Part print with two shaded views. Sizes in mm from the minimum x, y, z corner. Round coordinates to 2 decimals unless told otherwise and drop trailing zeros. Order: outer loops, then holes, each group sorted by start corner. A loop starts at its lowest first (then second) coordinate and runs counter-clockwise, first axis right, second up. Notation, with made-up numbers: M 64,16 L 71,16 A16 cw 71,30 Z; hole C 56,42.5 d1. An arc over 180 degrees is marked long. One line per question, with ' | ' between items. Start each with the question number.
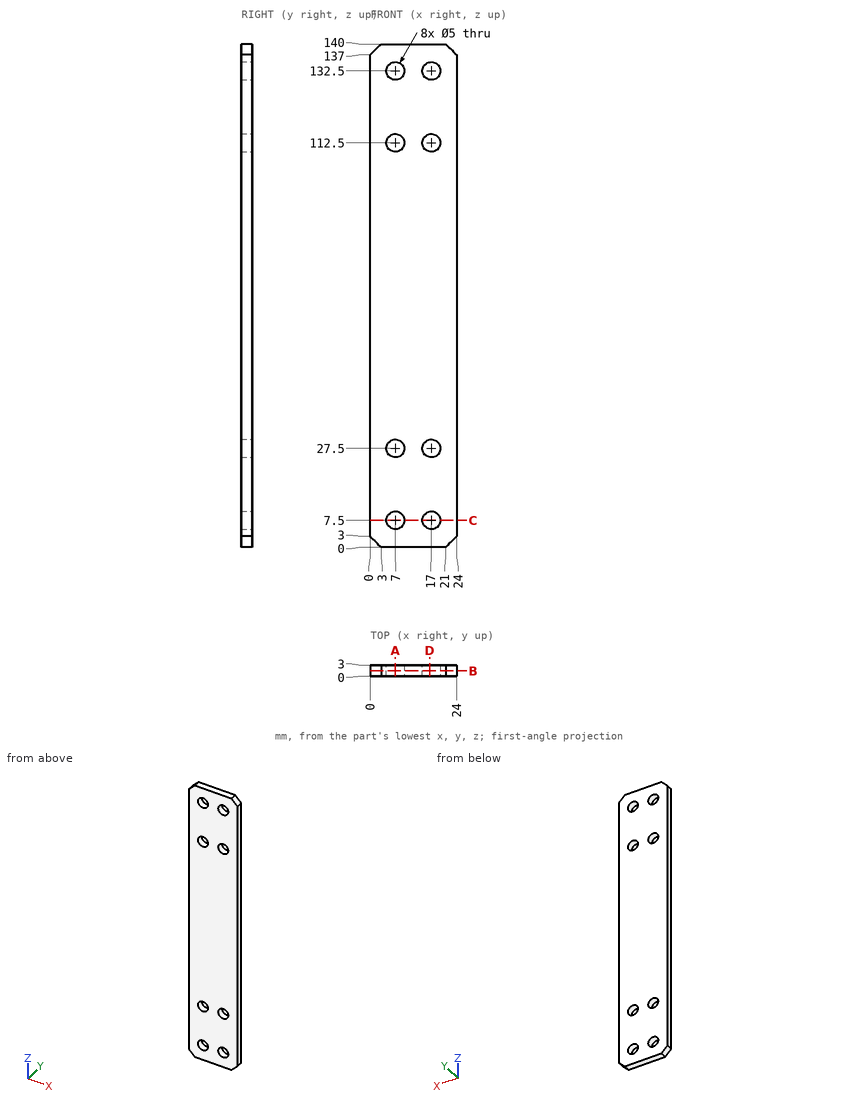
Item 1: Cut at D-D on x = 16.5. Write the cut outline in (y, z).
Item 2: Wall check: line 1 along X through (y, z) = (2.15, 27.5); line 2 along Z through (x, y) = (17, 0.65); line 3 along Z through (x, y) = (6.5, 1.6). Give the ranges that are in metal, low to high. Write a range as [from, to].
Item 3: Cut at C-C on z = 7.5. Write the cut outline in (x, y), then the cut area to 3 significant figures.
Item 4: Cut at B-B on y = 1.45. Count the separate pieces of the cut face and the enclosed holes in it, then the cut area to 3 significant figures.
Item 5: Cut at A-A on x = 7. Write the cut outline in (y, z), then the cut area to 3 significant figures.
Results found:
1) outline: M 0,0 L 3,0 L 3,5.05 L 0,5.05 Z; M 0,9.95 L 3,9.95 L 3,25.05 L 0,25.05 Z; M 0,29.95 L 3,29.95 L 3,110.05 L 0,110.05 Z; M 0,114.95 L 3,114.95 L 3,130.05 L 0,130.05 Z; M 0,134.95 L 3,134.95 L 3,140 L 0,140 Z
2) line 1: x = [0, 4.5], [9.5, 14.5], [19.5, 24] | line 2: z = [0, 5], [10, 25], [30, 110], [115, 130], [135, 140] | line 3: z = [0, 5.05], [9.95, 25.05], [29.95, 110.05], [114.95, 130.05], [134.95, 140]
3) outline: M 0,0 L 4.5,0 L 4.5,3 L 0,3 Z; M 9.5,0 L 14.5,0 L 14.5,3 L 9.5,3 Z; M 19.5,0 L 24,0 L 24,3 L 19.5,3 Z | area: 42.0 mm^2
4) separate pieces: 1 | enclosed holes: 8 | area: 3,180 mm^2
5) outline: M 0,0 L 3,0 L 3,5 L 0,5 Z; M 0,10 L 3,10 L 3,25 L 0,25 Z; M 0,30 L 3,30 L 3,110 L 0,110 Z; M 0,115 L 3,115 L 3,130 L 0,130 Z; M 0,135 L 3,135 L 3,140 L 0,140 Z | area: 360 mm^2
